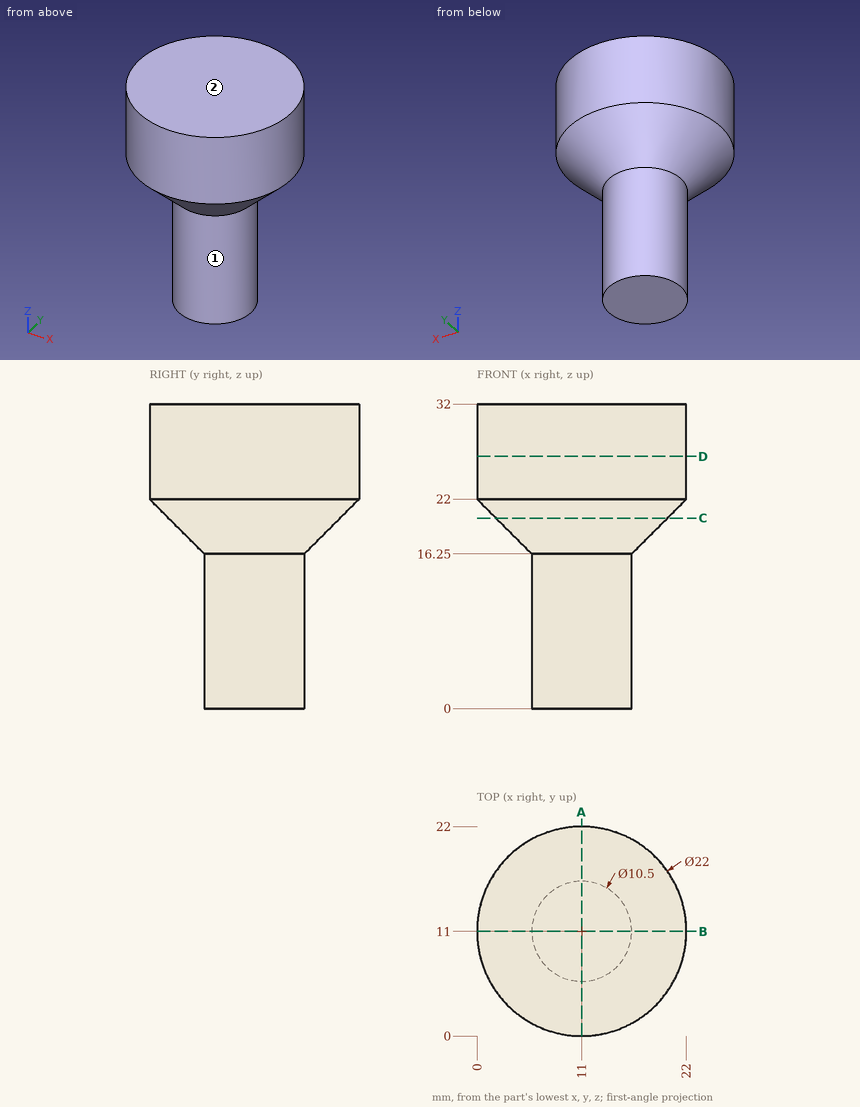
Design review of the part shown in the three views and the two pictorial views. Dimensions are in mm from the part's minimum x, y and z. A direction names the side the tool comes from. Give positions to 0.01 mm unless a question says otherwise; leave off trailing zeros. Write each loop counter-clockwise with the first axis right and the second up, starting at its lowest first coordinate (ties: lowest second). Pieces come first, ordered by that corner, then holes. Notation, with made-up numbers: M 18.25,-10.75 L 37.25,-10.75 A4 ccw 37.25,-6.75 Z; hole C -35.5,84.25 d6. An arc over 180 degrees is marked long. Answer in a Markdown table with one row per item.
Item 1: For P1, Ø4, axis at y = 3.5, z = 17.5, coming from the +X side; P2, Ø6, axis at x = 4.5, y = 3, coming from the -Z side; P3, Ø1, axis at x = 17, z = 23, coming from the -Y side, all flat-tipped, find the tip position at first contact; note any pin that passes through.
Check sheet entries:
| item | result |
|---|---|
| P1 | x = 16.09 |
| P2 | z = 18.31 |
| P3 | y = 1.47 |
Item 2: For line 1 along X through (y, z) = (15, 29); line 2 along X through (y, z) = (7, 2); line 3 along Z through (x, y) = (9.5, 21.25), list the stretches that pass through material, from the lowest coordinate up.
Check sheet entries:
| item | result |
|---|---|
| line 1 | 0.75 to 21.25 |
| line 2 | 7.6 to 14.4 |
| line 3 | 21.36 to 32 |
Item 3: Add section D-D on z = 26.5. Give the boundary of the cut face in (x, y), plus the area to 3 significant figures.
Check sheet entries:
| item | result |
|---|---|
| outline | C 11,11 d22 |
| area | 380 mm2 |
Item 4: Add section C-C on z = 20. Give the boundary of the cut face in (x, y).
Check sheet entries:
| item | result |
|---|---|
| outline | C 11,11 d18 |
Item 5: Tool access review of the marked faces 1 and 2: name each direction out of +Z, -Z, +X, -X, +Y, -Y from which nothing blocks a thin tool from reaching the whole face with its end or side.
Check sheet entries:
| item | result |
|---|---|
| face 1 | -Z |
| face 2 | +Z, +X, -X, +Y, -Y |
Item 6: Add section A-A on x = 11. Give the boundary of the cut face in (y, z).
Check sheet entries:
| item | result |
|---|---|
| outline | M 0,22 L 5.75,16.25 L 5.75,0 L 16.25,0 L 16.25,16.25 L 22,22 L 22,32 L 0,32 Z |
